from build123d import *

# Parameters (mm, degrees)
F0_R     = 9.375
F0_R_2   = 7.987
F1_DEPTH = 5.115
F0_R_3   = 6.945
F2_DEPTH = 0.5
F5_SIZE  = 0.3


with BuildPart() as f1:
    # F0 (on Front) → F1 (new body, symmetric)
    with BuildSketch(Plane.XZ):
        Circle(F0_R)
        Circle(F0_R_2, mode=Mode.SUBTRACT)
    extrude(amount=F1_DEPTH, both=True)

    # F0 (on Front) → F2 (join, symmetric)
    with BuildSketch(Plane.XZ):
        Circle(F0_R_2)
        Circle(F0_R_3, mode=Mode.SUBTRACT)
    extrude(amount=F2_DEPTH, both=True)

    # F3 (on Right) → F4 (revolve)
    with BuildSketch(Plane.YZ):
        Polygon((0.275, 9.77), (0.275, 9.375), (5.115, 9.375), (5.115, 9.77), (2.7, 12.195), align=None)
        Polygon((-5.115, 9.375), (-0.275, 9.375), (-0.275, 9.77), (-2.7, 12.195), (-5.115, 9.77), align=None)
    revolve(axis=Axis((0, -0.5, 0), (0, -1, 0)))

    # F5
    f5_edges = [f1.edges().sort_by_distance(p)[0] for p in [
        (-7.987, 5.115, 0),
        (-7.987, -5.115, 0),
    ]]
    chamfer(f5_edges, length=F5_SIZE)


solid = f1.part
Geometry: final body of the model. Coordinates: model frame, mm. A direction names the side the tool comes from. Give positions to 0.01 mm unless a question says otherwise; leave off trailing zeros. Write each loop counter-clockwise with the first axis right and the second up, starting at its lowest first coordinate (ties: lowest second). Pieces come first, ordered by that corner, then holes.
(1) Access query for faces 4 (the flat face through (7.2, 5.115, 4.4)), 5 (the flat face through (-2, 0.5, 7)), 6 (the conical face through (8.77, 0.39, 4.56)), 7 (the cylindrical face through (-5.887, -2.627, 5.398)), 8 (the cylindrical face through (-1.51, 0.01, -6.78)). Directions: +Z, -Z, +X, -X, +Y, -Y. A direction counts if a zero-diameter tool reaches every point of the face in a straight line with its end or side. Return the directions, or none.
(2) Ray query, line 1 (Z direction, x = 7, y = -3); line 2 (Y direction, x = -10, z = -6.75); line 3 (Z direction, x = 4.25, y = -4). Return the intervals inside material, ascending.
(3) First-contact query: P1, Ø3, axis at x = -2, y = 2, coming from the +Z side; P2, Ø2, axis at y = -1, z = -6.5, coming from the +X side; P3, Ø2, axis at x = 2, y = -1, coming from the +Z side. Flat tips, straight axial feed; report the tip coordinate or a pass-through.
(4) Cut plane C-C, the plane y = 3.5. Return loops of the section in (x, z), then the cut area to 3 significant figures.
(5) Cut plane D-D, the plane y = 1.75. Return loops of the section in (x, z) (3 decimals).
(6) Mould query, pull axis X, two halves, no side actions, for faces 1 (the cylindrical face through (8.66, 0, -3.59)), 2 (the flat face through (7.2, -5.115, -4.4)), 3 (the flat face through (-2, -0.5, 7)). Classes: released by +X, released by -X, zero draft, split by the parting line, or undercut.
Values follow:
1. face 4: +Z, -Z, +X, -X, +Y
1. face 5: +Y
1. face 6: none
1. face 7: -Y
1. face 8: +Y, -Y
2. line 1: z = -9.62 to -3.85, 3.85 to 9.62
2. line 2: y = -2.83 to -2.57, 2.57 to 2.83
2. line 3: z = -10.03 to -6.76, 6.76 to 10.03
3. P1: stops at z = 12.18
3. P2: stops at x = 9.65
3. P3: stops at z = 11.33
4. outline: circle Ø22.78 at (0, 0); hole circle Ø15.97 at (0, 0)
4. area: 207 mm2
5. outline: circle Ø22.49 at (0, 0); hole circle Ø15.974 at (0, 0)
6. face 1: split by the parting line
6. face 2: zero draft
6. face 3: undercut
